Input: part model. Units: mm. Frame: model coordinates. Face numbers are marked on the shaded views. A direction names the side the tool comes from. Round coordinates to 2 decimals unless told otherwise and drop trailing zeros. Loops run counter-clockwise (first coordinate to the right, second up) from the corner with the lowest first, then second, coordinate; pieces in that order, holes last.
1) Access query for the marked faces 4 and 5. Directions: +Z, -Z, +X, -X, +Y, -Y. A direction counts if a zero-diameter tool reaches every point of the face in a straight line with its end or side. Return the directions, or none.
2) Section C-C, the plane x = 0. Return loops of the section in (y, z), and give its area (3 significant figures).
3) First-contact query: pin 1 (3 mm diameter, centred on x = 7.5, y = -1.5, fed in from -Z); pin 2 (7 mm diameter, centred on x = 0, y = 0, fed in from -Z); pin 3 (10 mm diameter, centred on x = -6, y = 6, fed in from +Z). Flat tips, straight axial feed; report the tip coordinate or a pass-through.
4) Draft query along X for the marked faces 1, 2 and 3. Return one class per face: pulls with the +X half, pulls with the -X half, needs draft (parallel to the pull), parting line crosses it, or undercut.
5) Section B-B, the plane z = 14. Return loops of the section in (x, y), and give its area (3 significant figures).
6) Ray query, line 1 along X through (y, z) = (16.5, 12); line 2 along Y through (x, z) = (16.5, 21); line 3 along Z through (x, y) = (0, -22.7). Return the intervals inside material, ascending.
7) Section A-A, the plane y = 0. Return loops of the section in (x, z), and give its area (3 significant figures).
8) Section D-D, the plane z = 20.5. Return loops of the section in (x, y), and give its area (3 significant figures).
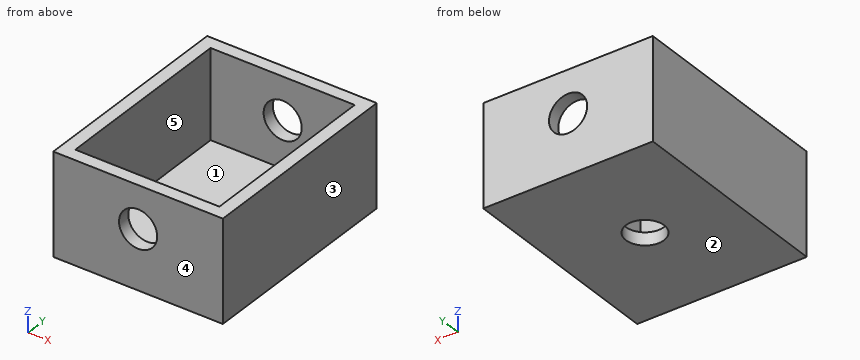
from build123d import *

# Parameters (mm, degrees)
F0_W     = 40
F0_H     = 50
F1_DEPTH = 24
F2_W     = 34
F2_H     = 44
F3_DEPTH = 21
F4_R     = 4.5
F5_DEPTH = 50.001
F6_R     = 4.5
F7_DEPTH = 3.001


with BuildPart() as f1:
    # F0 (on Top) → F1 (new body)
    with BuildSketch(Plane.XY):
        Rectangle(F0_W, F0_H)
    extrude(amount=F1_DEPTH)

    # F2 (on face) → F3 (cut, through all)
    with BuildSketch(Plane.XY.offset(24)):
        Rectangle(F2_W, F2_H)
    extrude(amount=-F3_DEPTH, mode=Mode.SUBTRACT)

    # F4 (on face) → F5 (cut, through all)
    with BuildSketch(Plane.XZ.offset(25)):
        with Locations((0, 14)):
            Circle(F4_R)
    extrude(amount=-F5_DEPTH, mode=Mode.SUBTRACT)

    # F6 (on face) → F7 (cut, through all)
    with BuildSketch(Plane.XY.offset(3)):
        Circle(F6_R)
    extrude(amount=-F7_DEPTH, mode=Mode.SUBTRACT)


solid = f1.part
Final values:
1. face 4: +Z, -Z, +X, -X, -Y
1. face 5: +Z
2. outline: (-25, 0) - (-4.5, 0) - (-4.5, 3) - (-22, 3) - (-22, 9.5) - (-25, 9.5) - close; (-25, 18.5) - (-22, 18.5) - (-22, 24) - (-25, 24) - close; (4.5, 0) - (25, 0) - (25, 9.5) - (22, 9.5) - (22, 3) - (4.5, 3) - close; (22, 18.5) - (25, 18.5) - (25, 24) - (22, 24) - close
2. area: 195 mm2
3. pin 1: stops at z = 0
3. pin 2: passes through
3. pin 3: stops at z = 3
4. face 1: undercut
4. face 2: needs draft
4. face 3: pulls with the +X half
5. outline: (-20, -25) - (-4.5, -25) - (-4.5, -22) - (-17, -22) - (-17, 22) - (-4.5, 22) - (-4.5, 25) - (-20, 25) - close; (4.5, -25) - (20, -25) - (20, 25) - (4.5, 25) - (4.5, 22) - (17, 22) - (17, -22) - (4.5, -22) - close
5. area: 450 mm2
6. line 1: x = -20 to -17, 17 to 20
6. line 2: y = -25 to -22, 22 to 25
6. line 3: z = 0 to 9.5, 18.5 to 24
7. outline: (-20, 0) - (-4.5, 0) - (-4.5, 3) - (-17, 3) - (-17, 24) - (-20, 24) - close; (4.5, 0) - (20, 0) - (20, 24) - (17, 24) - (17, 3) - (4.5, 3) - close
7. area: 219 mm2
8. outline: (-20, -25) - (20, -25) - (20, 25) - (-20, 25) - close; hole (-17, -22) - (17, -22) - (17, 22) - (-17, 22) - close
8. area: 504 mm2
